Design review of the part built by this model. Coordinates are the model's own, in mm. A direction names the side the tool comes from. Round coordinates to 2 decimals unless told otherwise and drop trailing zeros. Write each loop counter-clockwise with the first axis right and the second up, starting at its lowest first coordinate (ties: lowest second). Pieces come first, ordered by that corner, then holes. Notation, with made-up numbers: (-0.5, 55.5) - (9.5, 55.5) arc R24 ccw to (9.5, 66.5) - close; hole circle Ø7 at (-15, 63.5). An arc over 180 degrees is marked (long way). Use one line per item in the form item = value.
```python
from build123d import *

# Parameters (mm, degrees)
PAD008_DEPTH = 3
PAD009_DEPTH = 91
SKETCH019_R  = 2.5
PAD010_DEPTH = 5
SKETCH021_R  = 2.5
PAD011_DEPTH = 5


with BuildPart() as part:
    # Sketch017 → Pad008 (new body)
    with BuildSketch(Plane.XZ):
        Polygon((12.5, 2), (-12.5, 2), (-12.5, 18.5), (-8.5, 22.5), (8.5, 22.5), (12.5, 18.5), align=None)
    extrude(amount=PAD008_DEPTH)

    # Sketch018 → Pad009 (join)
    with BuildSketch(Plane.XZ):
        Polygon((-12.5, 2), (-12.5, 18.5), (-8.5, 22.5), (8.5, 22.5), (12.5, 18.5), (12.5, 2), (8.5, 2), (8.5, 18.5), (2, 18.5), (2, 2), (-2, 2), (-2, 18.5), (-8.5, 18.5), (-8.5, 2), align=None)
    extrude(amount=PAD009_DEPTH)

    # Sketch019 → Pad010 (join)
    with BuildSketch(Plane.XZ.offset(46)):
        Polygon((-12.5, 18.5), (-12.5, -19.5), (-8.5, -23.5), (8.5, -23.5), (12.5, -19.5), (12.5, 18.5), (8.5, 22.5), (-8.5, 22.5), align=None)
        with Locations((0, -3.5)):
            Circle(SKETCH019_R, mode=Mode.SUBTRACT)
    extrude(amount=PAD010_DEPTH)

    # Sketch021 → Pad011 (join)
    with BuildSketch(Plane.XZ.offset(91)):
        Polygon((-8.5, 22.5), (-12.5, 18.5), (-12.5, -19.5), (-8.5, -23.5), (8.5, -23.5), (12.5, -19.5), (12.5, 18.5), (8.5, 22.5), align=None)
        with Locations((0, -10.5)):
            Circle(SKETCH021_R, mode=Mode.SUBTRACT)
    extrude(amount=-PAD011_DEPTH)


with BuildPart() as part_1:
    # Body006 placement: moved
    add(part.part.moved(Location((0, -24, 0))))


solid = part_1.part
```
Q1. We need section B-B on x = 0. Write out the cut boundary in (y, z).
Calculated:
outline = (-115, -23.5) - (-110, -23.5) - (-110, -13) - (-115, -13) - close; (-115, -8) - (-110, -8) - (-110, 2) - (-75, 2) - (-75, -1) - (-70, -1) - (-70, 2) - (-24, 2) - (-24, 22.5) - (-115, 22.5) - close; (-75, -23.5) - (-70, -23.5) - (-70, -6) - (-75, -6) - close
Q2. Machinability: for faces 1 (the flat face through (0, -75, -7)), 2 (the flat face through (0, -47, 2)), 3 (the flat face through (0, -92, 2)), which of the approach directions +Z, -Z, +X, -X, +Y, -Y give a long, thin tool a straight path to every point of the face, cutting with its end or side? Answer none if there is none.
Calculated:
face_1 = -Z
face_2 = -Z, +X, -X, +Y
face_3 = -Z, +X, -X
Q3. For P1, Ø3, axis at x = 0.5, y = -93, coming from the -Z side; P2, Ø2, axis at x = -7, y = -56.5, coming from the -Z side; P3, Ø4.5, axis at x = 0, z = -10.5, coming from the -Y side, all flat-tipped, find the tip position at first contact; note any pin that passes through.
Calculated:
P1 = 2
P2 = 18.5
P3 = -75
Q4. To check wall thickness, follow line 1 along X through (y, z) = (-36, 11.5); line 2 along Y through (x, z) = (-7.75, 15.5); line 3 along Z through (x, y) = (0, -73.6). State the ranges of each line that lie inside material, in increasing order. Write a range as from..to.
Calculated:
line_1 = -12.5..-8.5, -2..2, 8.5..12.5
line_2 = -115..-110, -75..-70, -27..-24
line_3 = -23.5..-6, -1..22.5
Q5. We need section D-D on x = 9.5. Write out the cut boundary in (y, z).
Calculated:
outline = (-115, -22.5) - (-110, -22.5) - (-110, 2) - (-75, 2) - (-75, -22.5) - (-70, -22.5) - (-70, 2) - (-24, 2) - (-24, 21.5) - (-115, 21.5) - close
Q6. Draft analysis for pull direction Z (two halves, no side actions). For faces 4 (the flat face through (8.5, -92, 10)), 5 (the cylindrical face through (-0.54, -112.54, -12.94)), 6 (the flat face through (-5, -92, 18.5)), state which applies: released by +Z, released by -Z, zero draft, split by the parting line, or undercut.
Calculated:
face_4 = zero draft
face_5 = undercut
face_6 = released by -Z
Q7. We need section A-A on z = -12. Write out the cut boundary in (x, y), then the cut area to 3 significant figures.
Calculated:
outline = (-12.5, -115) - (-2, -115) - (-2, -110) - (-12.5, -110) - close; (-12.5, -75) - (12.5, -75) - (12.5, -70) - (-12.5, -70) - close; (2, -115) - (12.5, -115) - (12.5, -110) - (2, -110) - close
area = 230 mm2
Q8. We need section C-C on y = -45. Write out the cut boundary in (x, z), then the cut area to 3 significant figures.
Calculated:
outline = (-12.5, 2) - (-8.5, 2) - (-8.5, 18.5) - (-2, 18.5) - (-2, 2) - (2, 2) - (2, 18.5) - (8.5, 18.5) - (8.5, 2) - (12.5, 2) - (12.5, 18.5) - (8.5, 22.5) - (-8.5, 22.5) - (-12.5, 18.5) - close
area = 282 mm2
